Geometry: see drawing. Coordinates: mm, zero at the bounding-box minimum. A direction names the side the tool comes from. Coordinates: 2 decimals unless noted, no trailing zeros. Loops run counter-clockwise (first coordinate to the right, second up) from the corner with the lowest first, then second, coordinate; pieces in that order, holes last. Notation, with made-up numbers: (24.25, 0) - (72.25, 0) arc R24 cw to (72.25, 22) - close; hole circle Ø9 at (81.5, 22). An arc over 180 degrees is marked (long way). Write each question's results on one line, items separated by ' | '. Start each with the question number.
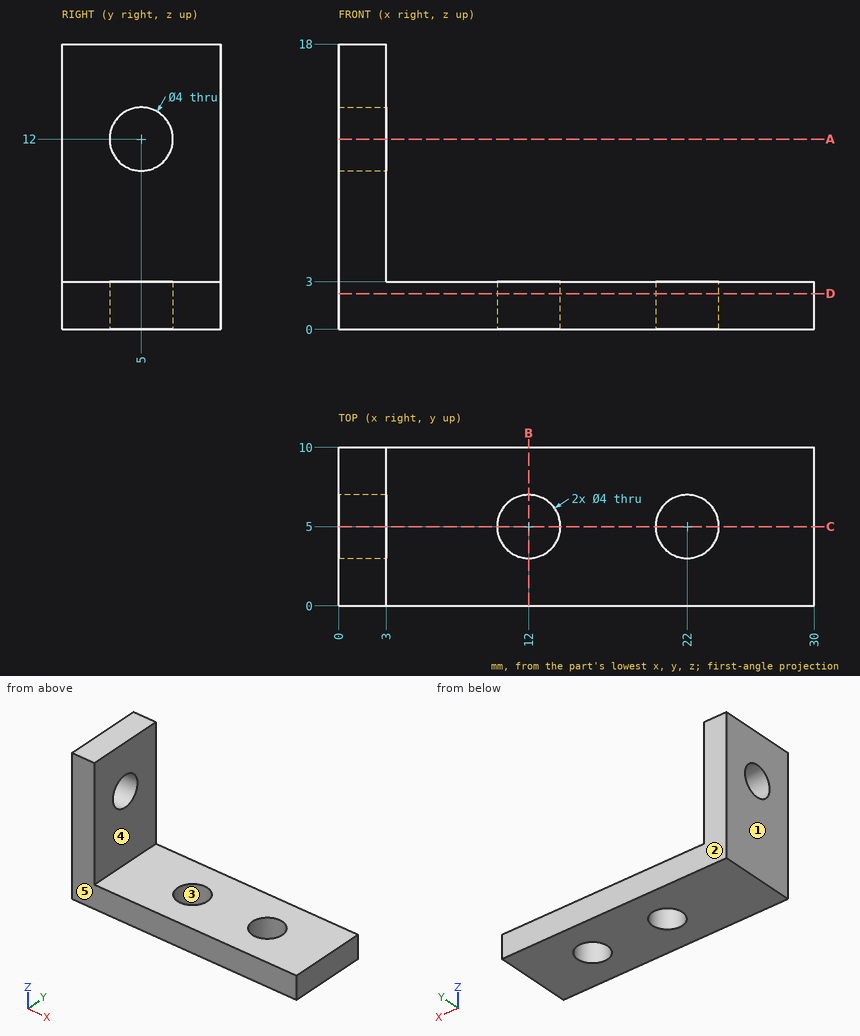
1) Section query D-D on z = 2.25. Output: boundary loops of the cut face in (x, y), and give its area (3 significant figures).
2) Pin query (flat end, axial travel): pin 1 Ø5 at (y, z) = (7, 14) entering from +X; pin 2 Ø1 at (x, z) = (23.5, 4.5) entering from -Y; pin 3 Ø5 at (x, y) = (18, 7.5) entering from +Z; pin 4 Ø5 at (x, y) = (22, 5) entering from -Z. Return the tip coordinate at first contact, or that it passes through.
3) Access query for the marked faces 4 and 5. Directions: +Z, -Z, +X, -X, +Y, -Y. A direction counts if a zero-diameter tool reaches every point of the face in a straight line with its end or side. Return the directions, or none.
4) Material intervals for line 1 (Z direction, x = 1.65, y = 5); line 2 (Y direction, x = 22, z = 1.95); line 3 (Z direction, x = 28.25, y = 4.25), sorted ascending. Write a range as [from, to].
5) Section query A-A on z = 12. Output: boundary loops of the cut face in (x, y).
6) Pull-direction query (X, two-part tool) for the marked faces 1, 2 and 3; classes: released by +X, released by -X, zero draft, split by the parting line, or undercut.
7) Section query B-B on x = 12. Output: boundary loops of the cut face in (y, z).
8) Section query C-C on y = 5. Output: boundary loops of the cut face in (x, z), and give its area (3 significant figures).
Returned:
1) outline: (0, 0) - (30, 0) - (30, 10) - (0, 10) - close; hole circle Ø4 at (12, 5); hole circle Ø4 at (22, 5) | area: 275 mm²
2) pin 1: stops at x = 3 | pin 2: passes through | pin 3: stops at z = 3 | pin 4: stops at z = 0
3) face 4: +Z, +X, +Y, -Y | face 5: +Z, -Z, +X, -X, -Y
4) line 1: z = [0, 10], [14, 18] | line 2: y = [0, 3], [7, 10] | line 3: z = [0, 3]
5) outline: (0, 0) - (3, 0) - (3, 3) - (0, 3) - close; (0, 7) - (3, 7) - (3, 10) - (0, 10) - close
6) face 1: released by -X | face 2: zero draft | face 3: undercut
7) outline: (0, 0) - (3, 0) - (3, 3) - (0, 3) - close; (7, 0) - (10, 0) - (10, 3) - (7, 3) - close
8) outline: (0, 0) - (10, 0) - (10, 3) - (3, 3) - (3, 10) - (0, 10) - close; (0, 14) - (3, 14) - (3, 18) - (0, 18) - close; (14, 0) - (20, 0) - (20, 3) - (14, 3) - close; (24, 0) - (30, 0) - (30, 3) - (24, 3) - close | area: 99.0 mm²
